Input: part model. Units: mm. Frame: model coordinates. A direction names the side the tool comes from. Coordinates: 2 decimals unless noted, no trailing zeros. Write each loop counter-clockwise with the first axis right and the second up, starting at its lowest first coordinate (ties: lowest second). Pieces come first, ordered by that corner, then holes. Notation, with made-up numbers: M 67,7 L 106,7 A24 ccw 106,26 Z; hole C -2.5,62.25 d4. An arc over 180 degrees is marked long. Use one line per item in the form item = value.
from build123d import *

# Parameters (mm, degrees)
SKETCH1_R               = 10
BOSS_EXTRUDE1_DEPTH     = 7
SKETCH2_R               = 10
BOSS_EXTRUDE2_DEPTH     = 1
SKETCH3_R               = 2.5
BOSS_EXTRUDE3_DEPTH     = 4
SKETCH4_R               = 1.5
CUT_EXTRUDE1_DEPTH      = 4
CUT_EXTRUDE2_DEPTH      = 2
CUT_EXTRUDE2_DEPTH_BACK = 20.397164741
SKETCH5_R               = 1.4


with BuildPart() as part:
    # Sketch1 → Boss-Extrude1 (new body)
    with BuildSketch(Plane(origin=(0, 0, 0), x_dir=(1, 0, 0), z_dir=(0, 1, 0))):
        with Locations(Location((0, 0, 0), (0, 0, 270))):
            Circle(SKETCH1_R)
        with BuildLine():
            Line((-1.322875656, 1.5), (1.322875656, 1.5))
            ThreePointArc((1.322875656, 1.5), (0, -2), (-1.322875656, 1.5))
        make_face(mode=Mode.SUBTRACT)
    extrude(amount=BOSS_EXTRUDE1_DEPTH)

    # Sketch2 → Boss-Extrude2 (add)
    with BuildSketch(Plane(origin=(0, 7, 0), x_dir=(1, 0, 0), z_dir=(0, 1, 0))):
        with Locations(Location((0, 0, 0), (0, 0, 270))):
            Circle(SKETCH2_R)
    extrude(amount=BOSS_EXTRUDE2_DEPTH)

    # Sketch3 → Boss-Extrude3 (add)
    with BuildSketch(Plane(origin=(0, 8, 0), x_dir=(1, 0, 0), z_dir=(0, 1, 0))):
        with Locations(Location((0, 0, 0), (0, 0, 270))):
            Circle(SKETCH3_R)
    extrude(amount=BOSS_EXTRUDE3_DEPTH)

    # Sketch4 → Cut-Extrude1 (cut)
    with BuildSketch(Plane(origin=(0, 8, 0), x_dir=(1, 0, 0), z_dir=(0, 1, 0))):
        with Locations(Location((6, 0, 0), (0, 0, 270))):
            Circle(SKETCH4_R)
        with Locations(Location((0, -6, 0), (0, 0, 270))):
            Circle(SKETCH4_R)
        with Locations(Location((-6, 0, 0), (0, 0, 270))):
            Circle(SKETCH4_R)
        with Locations(Location((0, 6, 0), (0, 0, 270))):
            Circle(SKETCH4_R)
    extrude(amount=-CUT_EXTRUDE1_DEPTH, mode=Mode.SUBTRACT)

    # Sketch5 → Cut-Extrude2 (cut, two sides: drawn at the far end of the back side and taken through both)
    with BuildSketch(Plane.XY.offset(-1.5).offset(-CUT_EXTRUDE2_DEPTH_BACK)):
        with Locations(Location((0, 3, 0), (0, 0, 199.106605351))):
            Circle(SKETCH5_R)
    extrude(amount=CUT_EXTRUDE2_DEPTH + CUT_EXTRUDE2_DEPTH_BACK, mode=Mode.SUBTRACT)


solid = part.part
(1) Section query D-D on z = 0. Return the cut outline in (x, y), plus the area to 3 significant figures.
Computed:
outline = M -10,0 L -2,0 L -2,7 L 2,7 L 2,0 L 10,0 L 10,8 L 7.5,8 L 7.5,4 L 4.5,4 L 4.5,8 L 2.5,8 L 2.5,12 L -2.5,12 L -2.5,8 L -4.5,8 L -4.5,4 L -7.5,4 L -7.5,8 L -10,8 Z
area = 128 mm^2
(2) Pull-direction query (X, two-part tool) for faces 1 (the cylindrical face through (0.07, 6.03, -7.5)), 2 (the cylindrical face through (-2.44, 9.97, -0.54)), 3 (the flat face through (2.4, 0, -0.1)); classes: pulls with the +X half, pulls with the -X half, needs draft (parallel to the pull), parting line crosses it, or undercut.
Computed:
face_1 = undercut
face_2 = parting line crosses it
face_3 = needs draft
(3) Section query A-A on y = 6. Return the cut outline in (x, z).
Computed:
outline = C 0,0 d20; hole C -6,0 d3; hole C 0,-6 d3; hole C 0,6 d3; hole M -1.32,-1.5 L 1.32,-1.5 A2 ccw long Z; hole C 6,0 d3
(4) First-contact query: pin 1 Ø4 at (x, z) = (6, 0) entering from +Y; pin 2 Ø0.6 at (x, z) = (1, -5.5) entering from +Y; pin 3 Ø5 at (x, y) = (3.5, 5) entering from +Z. Flat tips, straight axial feed; report the tip coordinate or a pass-through.
Computed:
pin_1 = 8
pin_2 = 4
pin_3 = 9.95
(5) Section query C-C on x = -5.25. Return the cut outline in (y, z).
Computed:
outline = M 0,-8.51 L 8,-8.51 L 8,-1.3 L 4,-1.3 L 4,1.3 L 8,1.3 L 8,8.51 L 0,8.51 Z
(6) Section query B-B on z = 6. Return the cut outline in (x, y).
Computed:
outline = M -8,0 L 8,0 L 8,8 L 1.5,8 L 1.5,4 L -1.5,4 L -1.5,8 L -8,8 Z
(7) Line query: probe 1 along X at (y, z) = (5.75, 0); probe 2 along X at (y, z) = (3.75, 0); probe 3 along Y at (x, z) = (6, -3.75). Output: solid intervals per line, ascending.
Computed:
probe_1 = -10 to -7.5, -4.5 to -2, 2 to 4.5, 7.5 to 10
probe_2 = -10 to -2, 2 to 10
probe_3 = 0 to 8
(8) Set-up query: faces 4 (the cylindrical face through (3, 3.94, 9.54)), 5 (the flat face through (-2, 8, 2)), 6 (the flat face through (0, 12, 0)), 7 (the cylindrical face through (-0.325, 1.638, -5.775)), 8 (the flat face through (0, 1, -1.5)). Return all of +Z, -Z, +X, -X, +Y, -Y with unobstructed straight access to the full face (end or side cutting, diameter ignored); none if empty.
Computed:
face_4 = +Y, -Y
face_5 = +Y
face_6 = +Z, -Z, +X, -X, +Y
face_7 = -Z
face_8 = -Y
